Model file for the job. Use its own axes, mm. Face numbers are marked on the shaded views. A direction names the side the tool comes from. Give positions to 0.01 mm unless a question says otherwise; leave off trailing zeros. Loops run counter-clockwise (first coordinate to the right, second up) from the corner with the lowest first, then second, coordinate; pieces in that order, holes last. Notation, with made-up numbers: M 67,38.25 L 74,38.25 A25 cw 74,60.25 Z; hole C 35.25,11 d9. An arc over 180 degrees is marked long. Answer in a Markdown table with one row per item.
Autodesk Inventor part; units mm, degrees
ref_plane "YZ Plane" through (0, 0, 0) normal (1, 0, 0) x (0, 1, 0)
ref_plane "XZ Plane" through (0, 0, 0) normal (0, 1, 0) x (-1, 0, 0)
ref_plane "XY Plane" through (0, 0, 0) normal (0, 0, 1) x (1, 0, 0)
sketch "Sketch1" plane through (0, 0, 0) normal (0, 1, 0) x (-1, 0, 0)
  circle A0 centre (26.875, 0) radius 1.5
  circle A1 centre (0, -26.875) radius 1.5
  circle A2 centre (-26.875, 0) radius 1.5
  circle A3 centre (0, 26.875) radius 1.5
  circle A4 centre (19.0035, 19.0035) radius 1.5
  circle A5 centre (19.0035, -19.0035) radius 1.5
  circle A6 centre (-19.0035, -19.0035) radius 1.5
  circle A7 centre (-19.0035, 19.0035) radius 1.5
  circle A8 centre (0, 0) radius 28.75
  circle A9 centre (0, 0) radius 30
  point P0 (-23.5374, 22.0452)
  dimension "d9" = 3
  dimension "d10" = 3
  dimension "d11" = 3
  dimension "d12" = 3
  dimension "d13" = 3
  dimension "d14" = 3
  dimension "d15" = 3
  dimension "d16" = 3
  dimension "d17" = 57.5
  dimension "d33" = 60
extrude "Extrusion1" add sketch "Sketch1" along normal blind 5 contours A8 | A9
sketch "Sketch2" plane through (0, 5, 0) normal (0, 1, 0) x (1, 0, 0)
  circle A0 centre (0, 0) radius 25
  line L0 (22.1416, 4) -> (20.8701, 4)
  line L1 (22.1416, -4) -> (20.8701, -4)
  arc A1 (24.6779, 4) -> (-17.6137, 17.7414) centre (0, 0) ccw
  arc A2 (-17.6137, -17.7414) -> (24.6779, -4) centre (0, 0) ccw
  line L2 (24.6779, -4) -> (22.1416, -4)
  line L3 (24.6779, 4) -> (22.1416, 4)
  line L4 (-15.5618, -16.2506) -> (-14.5332, -15.5032)
  line L5 (-19.2354, -9.0311) -> (-15.1903, -6.0922)
  line L6 (-15.1903, -6.0922) -> (-10.4881, -12.5643)
  line L7 (-10.4881, -12.5643) -> (-14.5332, -15.5032)
  line L8 (-22.316, -11.2693) -> (-20.2641, -9.7784)
  line L9 (-17.6137, -17.7414) -> (-15.5618, -16.2506)
  line L10 (-20.2641, -9.7784) -> (-19.2354, -9.0311)
  circle A3 centre (0, 22.5) radius 1.5
  line L11 (-10.4881, 12.5643) -> (-15.1903, 6.0922)
  line L12 (-14.5332, 15.5032) -> (-10.4881, 12.5643)
  line L13 (-15.5618, 16.2506) -> (-14.5332, 15.5032)
  line L14 (-15.1903, 6.0922) -> (-19.2354, 9.0311)
  line L15 (-20.2641, 9.7784) -> (-19.2354, 9.0311)
  line L16 (-17.6137, 17.7414) -> (-15.5618, 16.2506)
  line L17 (-23.5374, 22.0452) -> (-13.679, 22.0452) construction
  line L18 (-22.316, 11.2693) -> (-20.2641, 9.7784)
  arc A4 (-22.316, 11.2693) -> (-22.316, -11.2693) centre (0, 0) ccw
  line L19 (15.8701, -4) -> (20.8701, -4)
  circle A5 centre (18.2029, -13.2252) radius 1.5
  circle A6 centre (0, -22.5) radius 1.5
  circle A7 centre (18.2029, 13.2252) radius 1.5
  line L20 (20.8701, 4) -> (15.8701, 4)
  line L21 (15.8701, 4) -> (15.8701, -4)
  arc A8 (-13.5023, -14.7543) -> (19.5959, -4) centre (0, 0) ccw
  arc A9 (19.5959, 4) -> (-13.5023, 14.7543) centre (0, 0) ccw
  arc A10 (-18.2046, 8.2821) -> (-18.2046, -8.2821) centre (0, 0) ccw
  circle A11 centre (-22.5, 0) radius 1.5
  circle A12 centre (0, 0) radius 20
  circle A13 centre (-22.5, 0) radius 2.5
  circle A14 centre (0, -22.5) radius 2.5
  circle A15 centre (18.2029, -13.2252) radius 2.5
  circle A16 centre (18.2029, 13.2252) radius 2.5
  circle A17 centre (0, 22.5) radius 2.5
  point P0 (-28.2397, -15.5731)
  point P1 (-23.5374, -22.0452)
  dimension "d20" = 50
  dimension "d21" = 36
  dimension "d22" = 5
  dimension "d23" = 5
  dimension "d24" = 3
  dimension "d25" = 3
  dimension "d26" = 3
  dimension "d27" = 3
  dimension "d28" = 3
  dimension "d29" = 5
  dimension "d30" = 5
extrude "Extrusion2" cut sketch "Sketch2" against normal blind 3 contours A16 | A15 | A17 | A14 | A13 | A3 | A5 | A6 | A7 | A11
sketch "Sketch3" plane through (0, 0, 0) normal (0, -1, 0) x (1, 0, 0)
  circle A0 centre (0, 0) radius 20
  circle A1 centre (0, 0) radius 10
  circle A2 centre (0, 15.75) radius 2.5
  circle A3 centre (15.75, 0) radius 2.5
  line L0 (0, 0) -> (11.1369, 11.1369)
  line L1 (0, 0) -> (15.75, 0) construction
  circle A4 centre (11.1369, 11.1369) radius 2.5
  circle A5 centre (11.1369, -11.1369) radius 2.5
  circle A6 centre (-11.1369, -11.1369) radius 2.5
  circle A7 centre (-11.1369, 11.1369) radius 2.5
  circle A8 centre (-15.75, 0) radius 2.5
  circle A9 centre (0, -15.75) radius 2.5
  dimension "d34" = 40
  dimension "d35" = 20
  dimension "d37" = 5
  dimension "d38" = 5
  dimension "d39" = 45
  dimension "d40" = 5
  dimension "d41" = 5
  dimension "d42" = 5
  dimension "d43" = 5
  dimension "d44" = 5
  dimension "d45" = 5
extrude "Extrusion3" add sketch "Sketch3" along normal blind 5
properties part number "mountingPlate"
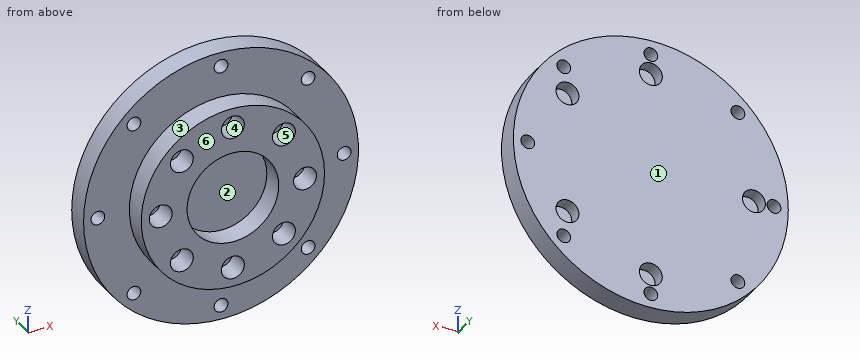
(1) Wall check: L1, parallel to Z at x = 0, y = -2.5; L2, parallel to Z at x = -1, y = 3.5; L3, parallel to Z at x = 1, y = -0.5. Give the ranges that are in metal, low to high.
Established:
| item | result |
|---|---|
| L1 | z = -20 to -18.25, -13.25 to -10, 10 to 13.25, 18.25 to 20 |
| L2 | z = -29.98 to -27.99, -25.76 to -24.79, -20.21 to 20.21, 24.79 to 25.76, 27.99 to 29.98 |
| L3 | z = -19.97 to -18.04, -13.46 to -9.95, 9.95 to 13.46, 18.04 to 19.97 |
(2) Which spindle directions (+Z, -Z, +X, -X, +Y, -Y) get a long thin tool onto all of the face, cutting with end or side? Do the marked faces 5 and 6. Say none if no direction does.
Established:
| item | result |
|---|---|
| face 5 | -Y |
| face 6 | +Z, -Z, +X, -X, -Y |
(3) Saw through at C-C, the plane x = -22.5. Give the cut face in (y, z), and give its area (3 significant figures).
Established:
| item | result |
|---|---|
| outline | M 0,-19.84 L 5,-19.84 L 5,-2.5 L 2,-2.5 L 2,2.5 L 5,2.5 L 5,19.84 L 0,19.84 Z |
| area | 183 mm2 |
(4) Saw through at B-B, the plane z = -22.5. Give the cut face in (x, y).
Established:
| item | result |
|---|---|
| outline | M -19.84,0 L 19.84,0 L 19.84,5 L 2.5,5 L 2.5,2 L -2.5,2 L -2.5,5 L -19.84,5 Z |
(5) Saw through at A-A, the plane y = -2.5. Count the separate pieces of the cut face and the enclosed holes in it, and give its area (3 significant figures).
Established:
| item | result |
|---|---|
| separate pieces | 1 |
| enclosed holes | 9 |
| area | 785 mm2 |
(6) Flat gauge pins, fed straight in: P1, Ø3, axis at x = -21.5, y = 1, coming from the +Z side; P2, Ø1, axis at x = 15.5, y = -2, coming from the +Z side; P3, Ø6, axis at x = 4.5, z = 0, coming from the -Y side; P4, Ø2.5, axis at x = -19, z = 19, coming from the -Y side. Where does each tip first touch, or does it go through?
Established:
| item | result |
|---|---|
| P1 | stops at z = 22.36 |
| P2 | stops at z = 13.23 |
| P3 | stops at y = 0 |
| P4 | passes through |
(7) Mould opens along Z. For the marked faces 1, 2, 3 and 4 say: pulls with the +Z half, pulls with the -Z half, needs draft (parallel to the pull), parting line crosses it, or undercut.
Established:
| item | result |
|---|---|
| face 1 | needs draft |
| face 2 | undercut |
| face 3 | parting line crosses it |
| face 4 | undercut |
